```python
from build123d import *

# Parameters (mm, degrees)
F0_W     = 825.5
F0_H     = 1930.4
F1_DEPTH = 19.05
F2_W     = 723.9
F2_H     = 1828.8
F3_DEPTH = 12.7


with BuildPart() as f1:
    # F0 (on Front) → F1 (new body)
    with BuildSketch(Plane.XZ):
        with Locations((412.75, 965.2)):
            Rectangle(F0_W, F0_H)
        Polygon((101.6, 185.164932), (101.6, 914.4), (101.6, 965.2), (101.6, 1016), (101.6, 1745.235068), (101.6, 1828.8), (165.579401, 1828.8), (723.9, 1828.8), (723.9, 1099.564932), (723.9, 1016), (723.9, 965.2), (723.9, 914.4), (723.9, 830.835068), (723.9, 101.6), (165.579401, 101.6), (101.6, 101.6), align=None, mode=Mode.SUBTRACT)
        Polygon((101.6, 1828.8), (101.6, 1745.235068), (659.920599, 1016), (723.9, 1016), align=None)
        Polygon((101.6, 1828.8), (723.9, 1016), (723.9, 1099.564932), (165.579401, 1828.8), align=None)
        Polygon((101.6, 1016), (101.6, 965.2), (723.9, 965.2), (723.9, 1016), (659.920599, 1016), align=None)
        Polygon((101.6, 965.2), (101.6, 914.4), (659.920599, 914.4), (723.9, 914.4), (723.9, 965.2), align=None)
        Polygon((659.920599, 914.4), (101.6, 185.164932), (101.6, 101.6), (723.9, 914.4), align=None)
        Polygon((723.9, 914.4), (101.6, 101.6), (165.579401, 101.6), (723.9, 830.835068), align=None)
    extrude(amount=F1_DEPTH)

    # F2 (on face) → F3 (join)
    with BuildSketch(Plane(origin=(0, 0, 0), x_dir=(-1, 0, 0), z_dir=(0, 1, 0))):
        with Locations((-412.75, 965.2)):
            Rectangle(F2_W, F2_H)
    extrude(amount=F3_DEPTH)


solid = f1.part
```
Could you check a few things on this model? Use its own coordinates, in mm. A direction names the side the tool comes from. Round coordinates to 2 decimals unless told otherwise and drop trailing zeros. Loops run counter-clockwise (first coordinate to the right, second up) from the corner with the lowest first, then second, coordinate; pieces in that order, holes last.
Q1. I want a section at C-C (x = 264). Write out the boundary of the cut face in (y, z), and give its area (3 significant figures).
Q2. On a 3-axis mill with a long thin cutter (end or side, diameter ignored), from which of +Z, -Z, +X, -X, +Y, -Y can I reach the whole of each face in a straight line? I mean faces 4 (the flat face through (448.648, -9.392, 1459.078)), 5 (the flat face through (418, 12.7, 978)). Say none if no direction works.
Q3. I want a section at B-B (z = 992.5). Write out the boundary of the cut face in (x, y).
Q4. Thinking about a two-plate mould opening in Z: for faces 1 (the flat face through (407, -19.05, 979)), 2 (the flat face through (384.67, -9.39, 554.89)), 3 (the flat face through (261, 0, 717)), which applies, pulls with the +Z half, pulls with the -Z half, needs draft (parallel to the pull), parting line crosses it, or undercut?
Q5. Please list where these lines run through material, in increasing order: L1, parallel to X at y = -17, z = 791; L2, parallel to Z at x = 688, y = -4; L3, parallel to Z at x = 450.5, y = -15.5.
Q6. I want a section at A-A (y = -9). Write out the boundary of the cut face in (x, z), and give its area (3 significant figures).
Q7. For P1, Ø8, axis at y = 4.5, z = 1200, coming from the -X side; P2, Ø6.5, axis at x = 550.5, y = 8, coming from the -Z side; P3, Ø3, axis at y = -10, z = 1636.5, coming from the -X side; P4, Ø5, axis at y = 3.5, z = 391.5, coming from the +X side, each with a flat end and sliding along its axis, tell me the tip position at first contact or that it passes through.
Q8. I want a section at D-D (z = 339.5). Write out the boundary of the cut face in (x, y).
Answer below:
1. outline: (-19.05, 0) - (0, 0) - (0, 50.8) - (12.7, 50.8) - (12.7, 1879.6) - (0, 1879.6) - (0, 1930.4) - (-19.05, 1930.4) - (-19.05, 1828.8) - (0, 1828.8) - (0, 1700.25) - (-19.05, 1700.25) - (-19.05, 1533.12) - (0, 1533.12) - (0, 1016) - (-19.05, 1016) - (-19.05, 914.4) - (0, 914.4) - (0, 397.28) - (-19.05, 397.28) - (-19.05, 230.15) - (0, 230.15) - (0, 101.6) - (-19.05, 101.6) - close
1. area: 35,400 mm2
2. face 4: -Y
2. face 5: +Z, -Z, +X, -X, +Y
3. outline: (0, -19.05) - (825.5, -19.05) - (825.5, 0) - (774.7, 0) - (774.7, 12.7) - (50.8, 12.7) - (50.8, 0) - (0, 0) - close
4. face 1: needs draft
4. face 2: undercut
4. face 3: undercut
5. L1: x = 0 to 101.6, 565.44 to 693.4, 723.9 to 825.5
5. L2: z = 0 to 101.6, 783.95 to 1146.45, 1828.8 to 1930.4
5. L3: z = 0 to 101.6, 473.74 to 640.87, 914.4 to 1016, 1289.53 to 1456.66, 1828.8 to 1930.4
6. outline: (0, 0) - (825.5, 0) - (825.5, 1930.4) - (0, 1930.4) - close; hole (101.6, 185.16) - (659.92, 914.4) - (101.6, 914.4) - close; hole (101.6, 1016) - (659.92, 1016) - (101.6, 1745.24) - close; hole (165.58, 101.6) - (723.9, 101.6) - (723.9, 830.84) - close; hole (165.58, 1828.8) - (723.9, 1099.56) - (723.9, 1828.8) - close
6. area: 779,000 mm2
7. P1: stops at x = 50.8
7. P2: stops at z = 50.8
7. P3: stops at x = 0
7. P4: stops at x = 774.7
8. outline: (0, -19.05) - (101.6, -19.05) - (101.6, 0) - (219.76, 0) - (219.76, -19.05) - (347.72, -19.05) - (347.72, 0) - (723.9, 0) - (723.9, -19.05) - (825.5, -19.05) - (825.5, 0) - (774.7, 0) - (774.7, 12.7) - (50.8, 12.7) - (50.8, 0) - (0, 0) - close
